Geometry check sheet. Reference: the model listing, model coordinates, mm. Give positions to 0.01 mm unless a question says otherwise; leave off trailing zeros. Order: outer loops, then holes, each group sorted by start corner. A loop starts at its lowest first (then second) coordinate and runs counter-clockwise, first axis right, second up. Notation, with made-up numbers: M 70.25,62.5 L 109.25,62.5 A16 cw 109.25,77.5 Z; hole C 22,-4 d7. An arc over 180 degrees is marked long. Answer as CSV lines item,"result".
from build123d import *

# Parameters (mm, degrees)
SKETCH1_W               = 160
SKETCH1_H               = 64.94
BOSS_EXTRUDE1_DEPTH     = 5
CUT_EXTRUDE1_DEPTH      = 87.482951499
CUT_EXTRUDE1_DEPTH_BACK = 87.482951499
SKETCH2_R               = 2.25


with BuildPart() as part:
    # Sketch1 → Boss-Extrude1 (new body)
    with BuildSketch(Plane.YZ):
        Rectangle(SKETCH1_W, SKETCH1_H)
    extrude(amount=BOSS_EXTRUDE1_DEPTH)

    # Sketch2 → Cut-Extrude1 (cut, two sides: drawn at the far end of the back side and taken through both)
    with BuildSketch(Plane.YZ.offset(5).offset(-CUT_EXTRUDE1_DEPTH_BACK)):
        with Locations(Location((-75, -27.47, 0), (0, 0, 270))):
            Circle(SKETCH2_R)
        with Locations(Location((75, 22.47, 0), (0, 0, 270))):
            Circle(SKETCH2_R)
    extrude(amount=CUT_EXTRUDE1_DEPTH + CUT_EXTRUDE1_DEPTH_BACK, mode=Mode.SUBTRACT)


solid = part.part
(1) Material ranges on line 1 (Y direction, x = 2.6, z = -27.47); line 2 (Z direction, x = 3.3, y = -75); line 3 (Y direction, x = 2.5, z = 22.47), recorded low to high.
The answers:
line 1,"y = -80 to -77.25, -72.75 to 80"
line 2,"z = -32.47 to -29.72, -25.22 to 32.47"
line 3,"y = -80 to 72.75, 77.25 to 80"
(2) Draft check along Z on faces 1 (the face through (0, -1, 0)), 2 (the face through (2, -1, 32.47)), 3 (the face through (2.5, -77.2, -27)). Enter one of: +Z half, -Z half, draft (parallel to the pull), parting line (faces both ways), or undercut.
The answers:
face 1,"draft"
face 2,"+Z half"
face 3,"undercut"
(3) Section check A-A on y = 75. Enter the section's corners in (x, z).
The answers:
outline,"M 0,-32.47 L 5,-32.47 L 5,20.22 L 0,20.22 Z; M 0,24.72 L 5,24.72 L 5,32.47 L 0,32.47 Z"
(4) Section check B-B on z = 22.47. Enter the section's corners in (x, y), then the cut area to 4 significant figures.
The answers:
outline,"M 0,-80 L 5,-80 L 5,72.75 L 0,72.75 Z; M 0,77.25 L 5,77.25 L 5,80 L 0,80 Z"
area,"777.5 mm2"
